Work out the finished part from the listing and answer in its coordinate system (mm). Face numbers are marked on the shaded views. A direction names the side the tool comes from. Coordinates: 2 decimals unless noted, no trailing zeros. Loops run counter-clockwise (first coordinate to the right, second up) from the corner with the lowest first, then second, coordinate; pieces in that order, holes last. Notation, with made-up numbers: M -12.5,70 L 10.5,70 A4 cw 10.5,75 Z; hole C 64,55.5 d11. An arc over 180 degrees is marked long. Write each question's results on one line, items separated by ' | '.
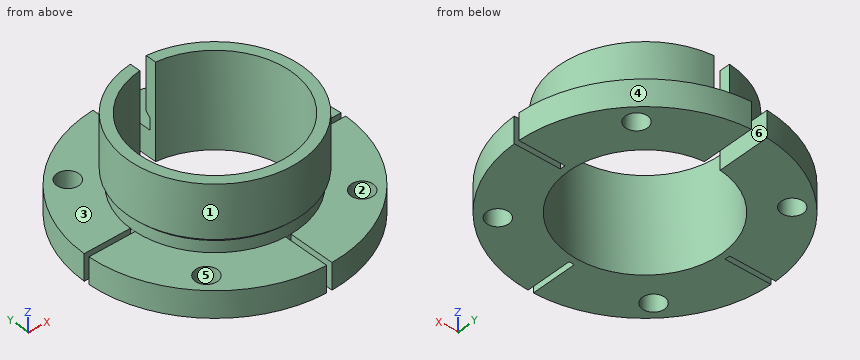
```python
from build123d import *

# Parameters (mm, degrees)
SKETCH001_W           = 3
SKETCH001_H           = 12
POCKET_DEPTH          = 18.001
SKETCH002_W           = 1
SKETCH002_H           = 8.8
POCKET001_DEPTH       = 5
POLARPATTERN_COUNT    = 4
SKETCH003_R           = 2.1
POCKET002_DEPTH       = 5
POLARPATTERN001_COUNT = 4


with BuildPart() as part:
    # Sketch → Revolution (revolve)
    with BuildSketch(Plane.XZ):
        Polygon((-14.5, 0), (-14.5, 18), (-16.5, 18), (-16.5, 8), (-15.7, 7.2), (-15.7, 5), (-24.5, 5), (-24.5, 0), align=None)
    revolve(axis=Axis((0, 0, 0), (0, 0, 1)))

    # Sketch001 → Pocket (cut, through all)
    with BuildSketch(Plane.XY.offset(18)):
        with Locations((0, 19.5)):
            Rectangle(SKETCH001_W, SKETCH001_H)
    extrude(amount=-POCKET_DEPTH, mode=Mode.SUBTRACT)

    # Sketch002 → Pocket001 (cut)
    with BuildSketch(Plane.XY):
        with Locations((0, -20.1)):
            Rectangle(SKETCH002_W, SKETCH002_H)
    pocket001 = extrude(amount=POCKET001_DEPTH, mode=Mode.SUBTRACT)

    # PolarPattern: Pocket001 ×4 about axis
    polarpattern_axis = Axis((0, 0, 0), (0, 0, 1))
    for i in range(1, POLARPATTERN_COUNT):
        add(pocket001.rotate(polarpattern_axis, i * 360 / POLARPATTERN_COUNT), mode=Mode.SUBTRACT)

    # Sketch003 → Pocket002 (cut)
    with BuildSketch(Plane.XY):
        with Locations((14.849242, 14.849242)):
            Circle(SKETCH003_R)
    pocket002 = extrude(amount=POCKET002_DEPTH, mode=Mode.SUBTRACT)

    # PolarPattern001: Pocket002 ×4 about axis
    polarpattern001_axis = Axis((0, 0, 0), (0, 0, 1))
    for i in range(1, POLARPATTERN001_COUNT):
        add(pocket002.rotate(polarpattern001_axis, i * 360 / POLARPATTERN001_COUNT), mode=Mode.SUBTRACT)


solid = part.part
```
1) Straight lines are drawn through the part: probe 1 along X at (y, z) = (0, 10); probe 2 along X at (y, z) = (-16.5, 3); probe 3 along Y at (x, z) = (15.5, 3). For each, find the intervals that lie inside material, in ascending order. Write a range as [from, to].
Check result:
probe 1: [-16.5, -14.5], [14.5, 16.5] | probe 2: [-18.11, -16.15], [-13.55, -0.5], [0.5, 13.55], [16.15, 18.11] | probe 3: [-18.97, -16.85], [-12.85, 12.85], [16.85, 18.97]
2) For a pull along X with two mould halves and no side action, classify the marked faces 1, 2, 3 and 4 as released by +X, released by -X, zero draft, split by the parting line, or undercut.
Check result:
face 1: split by the parting line | face 2: undercut | face 3: zero draft | face 4: released by +X
3) Which of the six approach directions +Z, -Z, +X, -X, +Y, -Y give full straight-line access (tool end or side, diameter ignored) to the marked faces 5 and 6?
Check result:
face 5: +Z, -Z | face 6: +Z, -Z, +Y
4) Find section A-A, the plane z = 6.5. Give the vertices of the cut face in (x, y), and give its area (3 significant figures).
Check result:
outline: M -1.5,14.42 L -1.5,15.63 A15.7 ccw long 1.5,15.63 L 1.5,14.42 A14.5 cw long Z | area: 110 mm^2
5) Find section B-B, the plane z = 14.75. Give the vertices of the cut face in (x, y).
Check result:
outline: M -1.5,14.42 L -1.5,16.43 A16.5 ccw long 1.5,16.43 L 1.5,14.42 A14.5 cw long Z
6) Given pin 1 Ø2 at (x, z) = (12, 3) entering from +Y; pin 2 Ø6 at (x, z) = (-1, 14.5) entering from -Y; pin 3 Ø2.5 at (x, y) = (14.85, -14.85) entering from +Z; pin 4 Ø5 at (x, y) = (-11, -17.5) entering from +Z, each flat-ended and moving along its own axis, determine where each tip first touches the part or whether it passes through.
Check result:
pin 1: y = 21.89 | pin 2: y = -16.5 | pin 3: through | pin 4: z = 5
